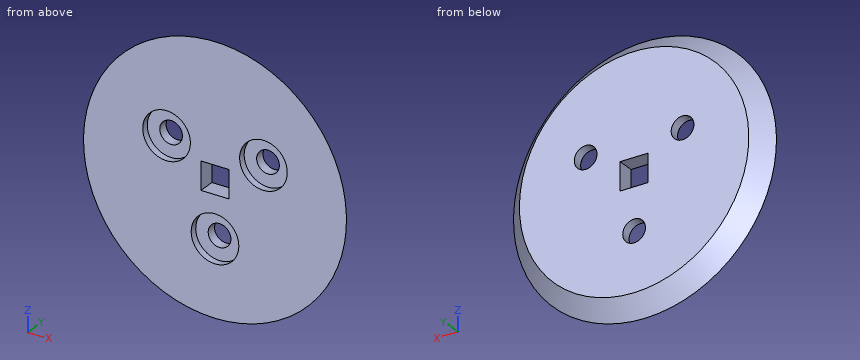
```python
from build123d import *

# Parameters (mm, degrees)
SKETCH1_R           = 31.75
SKETCH1_R_2         = 2.5796875
SKETCH1_W           = 6.35
SKETCH1_H           = 6.35
BOSS_EXTRUDE1_DEPTH = 3.81
CHAMFER1_SIZE       = 5.715
SKETCH2_R           = 5.409375008
CUT_EXTRUDE1_DEPTH  = 1.5875


with BuildPart() as part:
    # Sketch1 → Boss-Extrude1 (new body)
    with BuildSketch(Plane(origin=(0, 0, 0), x_dir=(1, 0, 0), z_dir=(0, 1, 0))):
        with Locations(Location((0, 0, 0), (0, 0, 90))):
            Circle(SKETCH1_R)
        with Locations(Location((0, 12.7, 0), (0, 0, 90))):
            Circle(SKETCH1_R_2, mode=Mode.SUBTRACT)
        with Locations(Location((10.998522628, -6.35, 0), (0, 0, 90))):
            Circle(SKETCH1_R_2, mode=Mode.SUBTRACT)
        with Locations(Location((-10.998522628, -6.35, 0), (0, 0, 90))):
            Circle(SKETCH1_R_2, mode=Mode.SUBTRACT)
        Rectangle(SKETCH1_W, SKETCH1_H, mode=Mode.SUBTRACT)
    extrude(amount=BOSS_EXTRUDE1_DEPTH)

    # Chamfer1
    # the kernel refuses this chamfer: 5.715 mm, written as the material it takes off along each edge
    with BuildSketch(Plane(origin=(0, 3.81, 0), x_dir=(0, 0, -1), z_dir=(1, 0, 0))) as chamfer1_piece_1:
        Polygon((31.75, -CHAMFER1_SIZE), (31.75 - CHAMFER1_SIZE, 0), (31.75, 0), align=None)
    revolve(axis=Axis((0, 3.81, 0), (0, 1, 0)), mode=Mode.SUBTRACT)

    # Sketch2 → Cut-Extrude1 (cut)
    with BuildSketch(Plane(origin=(0, 0, 0), x_dir=(-1, 0, 0), z_dir=(0, -1, 0))):
        with Locations(Location((0, 12.7, 0), (0, 0, 90))):
            Circle(SKETCH2_R)
        with Locations(Location((10.998522628, -6.35, 0), (0, 0, 90))):
            Circle(SKETCH2_R)
        with Locations(Location((-10.998522628, -6.35, 0), (0, 0, 90))):
            Circle(SKETCH2_R)
    extrude(amount=-CUT_EXTRUDE1_DEPTH, mode=Mode.SUBTRACT)


solid = part.part
```
Part model, mm, in its own coordinate system. Round coordinates to 2 decimals unless told otherwise and drop trailing zeros. Order: outer loops, then holes, each group sorted by start corner. A loop starts at its lowest first (then second) coordinate and runs counter-clockwise, first axis right, second up. Notation, with made-up numbers: M -6.5,19.5 L 20.5,19.5 A27 ccw 20.5,40.5 Z; hole C 32,87.5 d8. An arc over 180 degrees is marked long. Put each result on its own line as item: value. Start each with the question number.
1. Slice it at B-B on z = 0. List the corners of the cut face in (x, y) (3 decimals), then the cut area to 3 significant figures.
2. Slice it at D-D on z = 6.35. State how many separate pieces and enclosed holes the cut face has, then the cut area to 3 significant figures.
3. Drill centre lines: probe 1 along X at (y, z) = (2.65, 6.35); probe 2 along X at (y, z) = (1.25, 6.35); probe 3 along Z at (x, y) = (0.5, 1.05) (3 decimals). Where is each one in solid material? Low to high. Write a range as [from, to].
4. Slice it at C-C on y = 2.6. List the corners of the cut face in (x, z) (3 decimals).
5. Slice it at A-A on x = 0. List the corners of the cut face in (y, z) (1 decimal).
6. Drop flat-ended pins along their axis: pin 1 (6.5 mm diameter, centred on x = -11, z = 6.35, fed in from -Y); pin 2 (17.5 mm diameter, centred on x = -11, z = 6.35, fed in from -Y); pin 3 (1.9 mm diameter, centred on x = 0.5, y = 2.5, fed in from +Z); pin 4 (4 mm diameter, centred on x = 11, z = 6.35, fed in from +Y). Give the stop position or say it passes through.
Findings:
1. outline: M -29.845,0 L -3.175,0 L -3.175,3.81 L -26.035,3.81 Z; M 3.175,0 L 29.845,0 L 26.035,3.81 L 3.175,3.81 Z
1. area: 189 mm2
2. separate pieces: 3
2. enclosed holes: 0
2. area: 150 mm2
3. probe 1: [-26.44, -13.58], [-8.42, 8.42], [13.58, 26.44]
3. probe 2: [-27.88, -16.41], [-5.59, 5.59], [16.41, 27.88]
3. probe 3: [-28.791, -18.086], [-7.314, -3.175], [3.175, 28.791]
4. outline: C 0,0 d54.49; hole C -10.999,6.35 d5.159; hole M -3.175,-3.175 L 3.175,-3.175 L 3.175,3.175 L -3.175,3.175 Z; hole C 0,-12.7 d5.159; hole C 10.999,6.35 d5.159
5. outline: M 0,-29.8 L 3.8,-26 L 3.8,-15.3 L 1.6,-15.3 L 1.6,-18.1 L 0,-18.1 Z; M 0,-7.3 L 1.6,-7.3 L 1.6,-10.1 L 3.8,-10.1 L 3.8,-3.2 L 0,-3.2 Z; M 0,3.2 L 3.8,3.2 L 3.8,26 L 0,29.8 Z
6. pin 1: y = 1.59
6. pin 2: y = 0
6. pin 3: z = 28.29
6. pin 4: through
